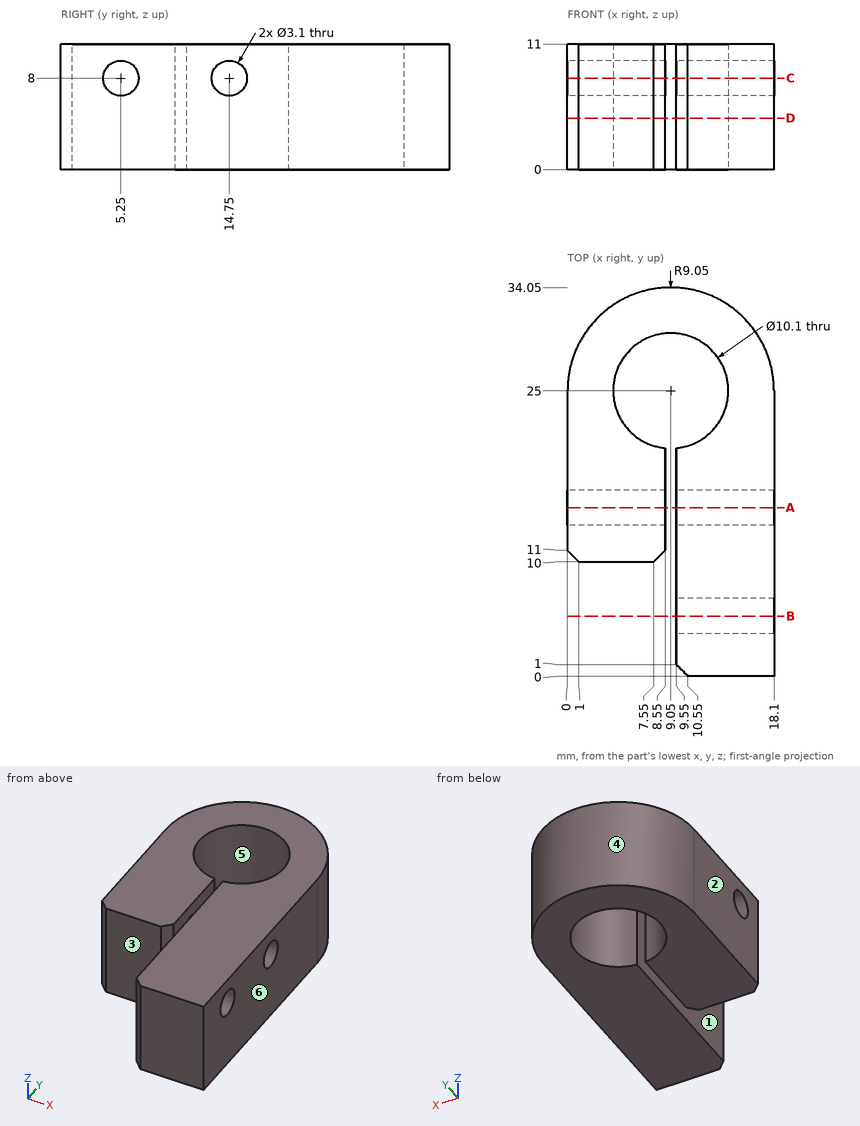
Can you work these out from the drawing? Everything is in mm from the part's minimum corner. A direction names the side the tool comes from. Give positions to 0.01 mm unless a question says otherwise; leave off trailing zeros. Loops run counter-clockwise (first coordinate to the right, second up) from the corner with the lowest first, then second, coordinate; pieces in that order, holes last. Notation, with made-up numbers: (39.25, 74.25) -> (46.25, 74.25) arc R4 cw to (46.25, 78.25) -> close; hole circle Ø7 at (-27, -39). An arc over 180 degrees is marked (long way). Return JSON: item names as keys, results as strings.
Q1. We'd pull the mould along Y, two halves only. Please class the marked faces 4, 5 and 6: released by +Y, released by -Y, zero draft, split by the parting line, or undercut.
Checks:
{"face 4": "released by +Y", "face 5": "undercut", "face 6": "zero draft"}
Q2. For pin 1 Ø1 at (y, z) = (28.5, 6.5) entering from +X; pin 2 Ø5 at (x, y) = (12, 18) entering from -Z; pin 3 Ø1.9 at (y, z) = (5.25, 8) entering from +X; pin 4 Ø2 at (x, z) = (4.5, 3) entering from -Y, each with a flat end and sliding along its axis, tell me the tip position at first contact or that it passes through.
Checks:
{"pin 1": "stops at x = 17.59", "pin 2": "stops at z = 0", "pin 3": "passes through", "pin 4": "stops at y = 10"}
Q3. On a 3-axis mill with a long thin cutter (end or side, diameter ignored), from which of +Z, -Z, +X, -X, +Y, -Y can I reach the whole of each face in a straight line? I mean the marked faces 1, 2 and 3. Say none if no direction works.
Checks:
{"face 1": "+Z, -Z, -Y", "face 2": "+Z, -Z, -X, +Y, -Y", "face 3": "+Z, -Z, -X, -Y"}
Q4. I need wall thicknesses on probe 1 along X at (y, z) = (15.5, 2.5); probe 2 along Z at (x, y) = (15.5, 14.75); probe 3 along Y at (x, z) = (15.25, 9.25). Which ranges of each line are inside material? Lowest first, please.
Checks:
{"probe 1": "x = 0 to 8.55, 9.55 to 18.1", "probe 2": "z = 0 to 6.45, 9.55 to 11", "probe 3": "y = 0 to 4.33, 6.17 to 13.83, 15.67 to 31.59"}
Q5. I want a section at D-D, the plane z = 4.5. List the corners of the cut face in (x, y) for me.
Checks:
{"outline": "(0, 11) -> (1, 10) -> (7.55, 10) -> (8.55, 11) -> (8.55, 19.97) arc R5.05 cw (long way) to (9.55, 19.97) -> (9.55, 1) -> (10.55, 0) -> (18.1, 0) -> (18.1, 25) arc R9.05 ccw to (0, 25) -> close"}
Q6. I want a section at C-C, the plane z = 8. List the corners of the cut face in (x, y) for me.
Checks:
{"outline": "(0, 11) -> (1, 10) -> (7.55, 10) -> (8.55, 11) -> (8.55, 13.2) -> (0, 13.2) -> close; (0, 16.3) -> (8.55, 16.3) -> (8.55, 19.97) arc R5.05 cw (long way) to (9.55, 19.97) -> (9.55, 16.3) -> (18.1, 16.3) -> (18.1, 25) arc R9.05 ccw to (0, 25) -> close; (9.55, 1) -> (10.55, 0) -> (18.1, 0) -> (18.1, 3.7) -> (9.55, 3.7) -> close; (9.55, 6.8) -> (18.1, 6.8) -> (18.1, 13.2) -> (9.55, 13.2) -> close"}
Q7. I want a section at A-A, the plane y = 14.75. List the corners of the cut face in (x, z) for me.
Checks:
{"outline": "(0, 0) -> (8.55, 0) -> (8.55, 6.45) -> (0, 6.45) -> close; (0, 9.55) -> (8.55, 9.55) -> (8.55, 11) -> (0, 11) -> close; (9.55, 0) -> (18.1, 0) -> (18.1, 6.45) -> (9.55, 6.45) -> close; (9.55, 9.55) -> (18.1, 9.55) -> (18.1, 11) -> (9.55, 11) -> close"}
Q8. I want a section at B-B, the plane y = 5.25. List the corners of the cut face in (x, z) for me.
Checks:
{"outline": "(9.55, 0) -> (18.1, 0) -> (18.1, 6.45) -> (9.55, 6.45) -> close; (9.55, 9.55) -> (18.1, 9.55) -> (18.1, 11) -> (9.55, 11) -> close"}
